```python
from build123d import *

# Parameters (mm, degrees)
BOSS_EXTRUDE1_DEPTH = 10
SKETCH1_3_R         = 4.45
BOSS_EXTRUDE2_DEPTH = 10


with BuildPart() as part:
    # Sketch1 → Boss-Extrude1 (new body)
    with BuildSketch(Plane(origin=(0, 0, 0), x_dir=(0, 0, -1), z_dir=(1, 0, 0))):
        with BuildLine():
            Line((1.303840481, 1.45), (-1.303840481, 1.45))
            ThreePointArc((-1.303840481, 1.45), (-0.793728878, -1.78114976), (1.95, 0))
            ThreePointArc((1.95, 0), (1.78114976, 0.793728878), (1.303840481, 1.45))
        make_face()
    extrude(amount=BOSS_EXTRUDE1_DEPTH)

    # Sketch1<3> → Boss-Extrude2 (add)
    with BuildSketch(Plane(origin=(0, 0, 0), x_dir=(0, 0, -1), z_dir=(1, 0, 0))):
        Circle(SKETCH1_3_R)
    extrude(amount=-BOSS_EXTRUDE2_DEPTH)


solid = part.part
```
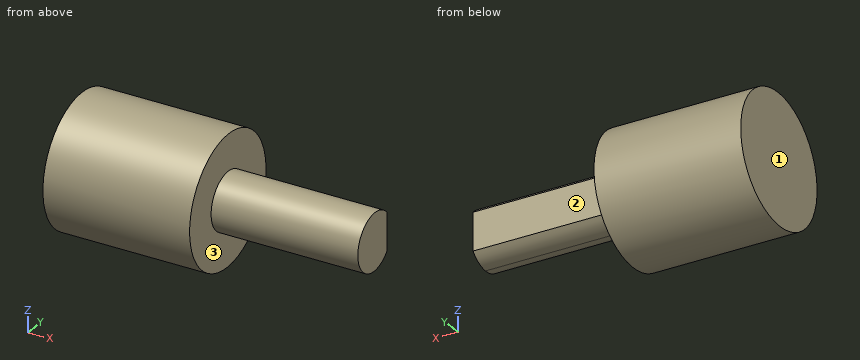
CAD build for the part. Positions are in the model's coordinates, mm. Face numbers are marked on the shaded views. A direction names the side the tool comes from. Give positions to 0.01 mm unless a question says otherwise; leave off trailing zeros. Order: outer loops, then holes, each group sorted by start corner. A loop starts at its lowest first (then second) coordinate and runs counter-clockwise, first axis right, second up.
(1) Saw through at D-D, the plane x = 1.75. Give the cut face in (y, z).
(2) Saw through at A-A, the plane z = 0. Give the cut face in (x, y), then the cut area to 3 significant figures.
(3) Flat gauge pins, fed straight in: pin 1 (1.5 mm diameter, centred on x = 2.5, y = 1.5, fed in from -Z); pin 2 (2 mm diameter, centred on x = 6, z = -3.5, fed in from +Y); pin 3 (2 mm diameter, centred on x = 5, z = 0, fed in from +Y). Where does each tip first touch, or does it go through?
(4) Tool access for the marked faces 1, 2 and 3: list every direction of +Z, -Z, +X, -X, +Y, -Y with a clear straight run to the whole face (end or side of a thin tool).
(5) Drill centre lines: L1, parallel to X at y = 2, z = 2.75; L2, parallel to Y at x = 9, z = 0; L3, parallel to Y at x = 2.25, z = -1.25. Where is each one in solid material? Low to high.
(6) Saw through at B-B, the plane y = 1. Give the cut face in (x, z).
(7) Saw through at C-C, the plane x = -8. Give the cut face in (y, z), then the cut area to 3 significant figures.
Results found:
1. outline: (1.45, -1.3) - (1.45, 1.3) arc R1.95 ccw (long way) to start
2. outline: (-10, -4.45) - (0, -4.45) - (0, -1.95) - (10, -1.95) - (10, 1.45) - (0, 1.45) - (0, 4.45) - (-10, 4.45) - close
2. area: 123 mm2
3. pin 1: stops at z = -1.8
3. pin 2: passes through
3. pin 3: stops at y = 1.45
4. face 1: +Z, -Z, -X, +Y, -Y
4. face 2: +Z, -Z, +X, +Y
4. face 3: +X
5. L1: x = -10 to 0
5. L2: y = -1.95 to 1.45
5. L3: y = -1.5 to 1.45
6. outline: (-10, -4.34) - (0, -4.34) - (0, -1.67) - (10, -1.67) - (10, 1.67) - (0, 1.67) - (0, 4.34) - (-10, 4.34) - close
7. outline: circle Ø8.9 at (0, 0)
7. area: 62.2 mm2
